from build123d import *

# Parameters (mm, degrees)
SKETCH1_W           = 12.7
SKETCH1_H           = 12.7
BOSS_EXTRUDE1_DEPTH = 80
SKETCH2_R           = 2
CUT_EXTRUDE1_DEPTH  = 82.991341006
CUT_EXTRUDE2_DEPTH  = 82.991341006
BOSS_EXTRUDE2_START = 17
SKETCH5_R           = 2
BOSS_EXTRUDE2_DEPTH = 17
SKETCH6_R           = 2
BOSS_EXTRUDE3_DEPTH = 17
SKETCH7_R           = 50
BOSS_EXTRUDE4_DEPTH = 2


with BuildPart() as part:
    # Sketch1 → Boss-Extrude1 (new body)
    with BuildSketch(Plane.XY):
        with Locations((6.35, 6.35)):
            Rectangle(SKETCH1_W, SKETCH1_H)
    extrude(amount=BOSS_EXTRUDE1_DEPTH)

    # Sketch2 → Cut-Extrude1 (cut, through all)
    with BuildSketch(Plane(origin=(0, 12.7, 0), x_dir=(1, 0, 0), z_dir=(0, 1, 0))):
        with Locations(Location((6.668720536, -5, 0), (0, 0, 270))):
            Circle(SKETCH2_R)
        with Locations(Location((6.668720536, -20, 0), (0, 0, 270))):
            Circle(SKETCH2_R)
        with Locations(Location((6.668720536, -60, 0), (0, 0, 270))):
            Circle(SKETCH2_R)
        with Locations(Location((6.668720536, -75, 0), (0, 0, 270))):
            Circle(SKETCH2_R)
    extrude(amount=-CUT_EXTRUDE1_DEPTH, mode=Mode.SUBTRACT)

    # Sketch4 → Cut-Extrude2 (cut, through all)
    with BuildSketch(Plane.ZY):
        with BuildLine():
            ThreePointArc((40, 2.727500863), (49.05, 6.35), (40, 9.972499137))
            ThreePointArc((40, 9.972499137), (30.95, 6.35), (40, 2.727500863))
        make_face()
    extrude(amount=-CUT_EXTRUDE2_DEPTH, mode=Mode.SUBTRACT)

    # Sketch5 → Boss-Extrude2 (add)
    with BuildSketch(Plane(origin=(0, 0, 0), x_dir=(1, 0, 0), z_dir=(0, 1, 0)).offset(BOSS_EXTRUDE2_START)):
        with Locations(Location((6.668720536, -20, 0), (0, 0, 270))):
            Circle(SKETCH5_R)
        with Locations(Location((6.668720536, -5, 0), (0, 0, 270))):
            Circle(SKETCH5_R)
    extrude(amount=-BOSS_EXTRUDE2_DEPTH)

    # Sketch6 → Boss-Extrude3 (add)
    with BuildSketch(Plane(origin=(0, 12.7, 0), x_dir=(1, 0, 0), z_dir=(0, 1, 0))):
        with Locations(Location((6.668720536, -75, 0), (0, 0, 270))):
            Circle(SKETCH6_R)
        with Locations(Location((6.668720536, -60, 0), (0, 0, 270))):
            Circle(SKETCH6_R)
    extrude(amount=-BOSS_EXTRUDE3_DEPTH)

    # Sketch7 → Boss-Extrude4 (add)
    with BuildSketch(Plane(origin=(0, 17, 0), x_dir=(1, 0, 0), z_dir=(0, 1, 0))):
        with Locations(Location((6.35, -40, 0), (0, 0, 270))):
            Circle(SKETCH7_R)
    extrude(amount=BOSS_EXTRUDE4_DEPTH)


solid = part.part
Check sheet for the modelled part. Datum: model origin and axes. Units: mm. A direction names the side the tool comes from. Coordinates: 2 decimals unless noted, no trailing zeros. Write each loop counter-clockwise with the first axis right and the second up, starting at its lowest first coordinate (ties: lowest second). Pieces come first, ordered by that corner, then holes.
Item 1: Depth check by flat-ended pin: pin 1 Ø5 at (y, z) = (11, 73) entering from -X; pin 2 Ø6.5 at (x, y) = (5.5, 7.5) entering from -Z; pin 3 Ø8.5 at (y, z) = (6.35, 43.8) entering from -X; pin 4 Ø6.5 at (x, y) = (6.5, 6) entering from +Z. Enter the tip coordinate at first touch or a pass-through.
Numbers:
pin 1: stops at x = 0
pin 2: stops at z = 0
pin 3: passes through
pin 4: stops at z = 80
Item 2: Scan lines: probe 1 along Y at (x, z) = (5, 43.8); probe 2 along Z at (x, y) = (5.75, 6.35); probe 3 along Y at (x, z) = (12, 37). Record each from-to range of solid material in increasing order.
Numbers:
probe 1: y = 0 to 1.1, 11.6 to 12.7, 17 to 19
probe 2: z = 0 to 30.95, 49.05 to 80
probe 3: y = 0 to 1.16, 11.54 to 12.7, 17 to 19
Item 3: Mould release check, pull along Z, two halves, no side actions. Record for faces 6 (the face through (6, 6, 0)), 7 (the face through (12.7, 2, 39.4)), 8 (the face through (6.261, 6.525, 30.953)): released by +Z, released by -Z, zero draft, split by the parting line, or undercut.
Numbers:
face 6: released by -Z
face 7: zero draft
face 8: undercut
Item 4: Cross-section at B-B on y = 8.5. Record the boundary of the cut face in (x, z).
Numbers:
outline: (0, 0) - (12.7, 0) - (12.7, 31.41) - (0, 31.41) - close; (0, 48.59) - (12.7, 48.59) - (12.7, 80) - (0, 80) - close
Item 5: Access from +Z, -Z, +X, -X, +Y, -Y to the whole of each face (thin tool, end or side, straight path). Record for faces 1 (the face through (7, 19, 39)), 2 (the face through (6.757, -2.12, 58.002)), 3 (the face through (0, 2, 39.4)), 4 (the face through (5.452, 14.88, 18.413)), 5 (the face through (6, 6, 80)).
Numbers:
face 1: +Z, -Z, +X, -X, +Y
face 2: -Y
face 3: +Z, -Z, -X, -Y
face 4: none
face 5: +Z, +X, -X, -Y
Item 6: Cross-section at A-A on z = 16. Record the boundary of the cut face in (x, y), then the cut area to 3 significant figures.
Numbers:
outline: (-37.51, 17) - (50.21, 17) - (50.21, 19) - (-37.51, 19) - close; (0, 0) - (12.7, 0) - (12.7, 12.7) - (0, 12.7) - close
area: 337 mm2
Item 7: Cross-section at C-C on z = 43.8. Record the boundary of the cut face in (x, y).
Numbers:
outline: (-43.51, 17) - (56.21, 17) - (56.21, 19) - (-43.51, 19) - close; (0, 0) - (12.7, 0) - (12.7, 1.1) - (0, 1.1) - close; (0, 11.6) - (12.7, 11.6) - (12.7, 12.7) - (0, 12.7) - close
Item 8: Cross-section at D-D on z = 75. Record the boundary of the cut face in (x, y), then the cut area to 3 significant figures.
Numbers:
outline: (-29.36, 17) - (42.06, 17) - (42.06, 19) - (-29.36, 19) - close; (0, 0) - (4.67, 0) - (4.67, -4.3) - (8.67, -4.3) - (8.67, 0) - (12.7, 0) - (12.7, 12.7) - (0, 12.7) - close
area: 321 mm2
